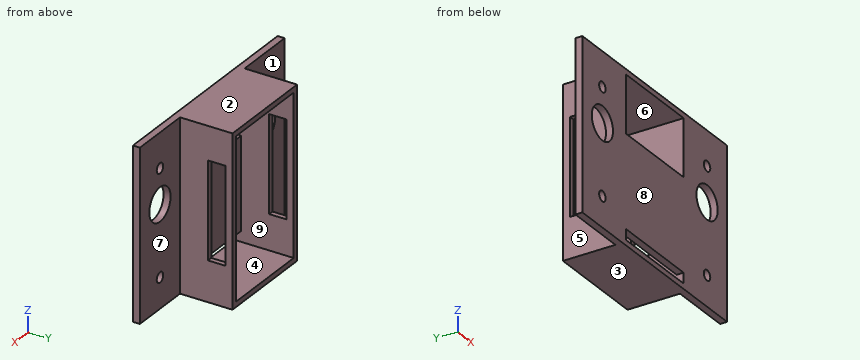
Autodesk Inventor part; units mm, degrees
ref_plane "Work Plane1" through (-23.6, 15, -43.3) normal (0, 1, 0) x (0, 0, 1)
ref_plane "YZ Plane" through (0, 0, 0) normal (1, 0, 0) x (0, 1, 0)
ref_plane "XZ Plane" through (0, 0, 0) normal (0, 1, 0) x (-1, 0, 0)
sketch "Sketch1" plane through (0, 0, 0) normal (0, 1, 0) x (-1, 0, 0)
  line L0 (0, 0) -> (26, 0)
  line L1 (26, 0) -> (26, -45.5)
  line L2 (26, -45.5) -> (0, -45.5)
  line L3 (0, -45.5) -> (0, 0)
  line L4 (-1.5, 0) -> (-1.5, -45.5)
  line L5 (-1.5, -45.5) -> (-1.5, -47)
  line L6 (-1.5, -47) -> (26, -47)
  line L7 (26, -47) -> (27.5, -47)
  line L8 (27.5, -47) -> (27.5, 0)
  line L9 (27.5, 0) -> (27.5, 1.5)
  line L10 (27.5, 1.5) -> (-1.5, 1.5)
  line L11 (-1.5, 1.5) -> (-1.5, 0)
  dimension "d0" = 26
  dimension "d1" = 45.5
  dimension "d3" = 1.5
  dimension "d4" = 1.5
  dimension "d5" = 1.5
extrude "Extrusion1" add sketch "Sketch1" along normal blind 15
sketch "Sketch2" plane through (1.5, 0, 1.5) normal (1, 0, 0) x (0, 0, -1)
  line L0 (9.5, 13) -> (37, 13)
  line L1 (37, 13) -> (37, 8)
  line L2 (9.5, 13) -> (9.5, 8)
  line L3 (37, 8) -> (9.5, 8)
  point P0 (1.5, 0)
  point P1 (48.5, 0)
extrude "Extrusion2" cut sketch "Sketch2" against normal up to surface (29 mm away)
sketch "Sketch3" plane through (0, 0, 0) normal (0, -1, 0) x (1, 0, 0)
  line L0 (1.5, 1.5) -> (1.5, -47)
  line L1 (-27.5, 1.5) -> (1.5, 1.5)
  line L2 (-27.5, -47) -> (-27.5, 1.5)
  line L3 (1.5, -47) -> (-27.5, -47)
  line L4 (0, 0) -> (-26, 0)
  line L5 (0, -45.5) -> (0, 0)
  line L6 (-26, -45.5) -> (0, -45.5)
  line L7 (-26, 0) -> (-26, -45.5)
  line L8 (0, 0) -> (-26, 0)
  line L9 (-26, 0) -> (-26, -3)
  line L10 (-26, 0) -> (-26, -45.5)
  line L11 (-26, -3) -> (0, -3)
  line L12 (0, -45.5) -> (0, 0)
  line L13 (-26, -45.5) -> (-26, -42.5)
  line L14 (-26, -42.5) -> (0, -42.5)
  line L15 (0, -42.5) -> (-26, -42.5)
  line L16 (-26, -42.5) -> (-26, -3)
  line L17 (-26, -3) -> (0, -3)
  line L18 (0, -3) -> (0, -42.5)
  dimension "d15" = 3
  dimension "d16" = 3
extrude "Extrusion3" add sketch "Sketch3" along normal blind 2 contours L0 L3 L2 L1 | L5 L14 L7 L11
sketch "Sketch5" plane through (0, -2, 0) normal (0, -1, 0) x (1, 0, 0)
  line L0 (0, -3) -> (-26, -3)
  line L1 (0, -35.5) -> (0, -8)
  line L2 (-26, -3) -> (0, -3)
  line L3 (0, -3) -> (0, -16.2813)
  line L4 (0, -16.2813) -> (-26, -16.2813)
  line L5 (-26, -16.2813) -> (-26, -3)
  point P0 (0, 0)
  point P1 (0, -8)
ref_plane "Work Plane1" through (-23.6, 15, -43.3) normal (0, 1, 0) x (0, 0, 1)
extrude "Extrusion4" cut sketch "Sketch5" against normal up to surface (17 mm away)
sketch "Sketch6" plane through (1.5, 15, 1.5) normal (1, 0, 0) x (0, 0, -1)
  line L0 (0, -17) -> (48.5, -17)
  line L1 (0, -17) -> (0, -15)
  line L2 (0, 0) -> (0, -17)
  line L3 (0, -15) -> (48.5, -15)
  line L4 (48.5, -17) -> (48.5, 0)
  line L5 (48.5, -17) -> (48.5, -15)
  line L6 (48.5, -17) -> (0, -17)
  point P0 (1.5, -15)
  dimension "d21" = 2
extrude "Extrusion5" add sketch "Sketch6" along normal blind 18
sketch "Sketch7" plane through (-27.5, 15, -47) normal (-1, 0, 0) x (0, 0, 1)
  line L0 (0, -15) -> (48.5, -15)
  line L1 (48.5, -15) -> (48.5, -17)
  line L2 (48.5, -17) -> (0, -17)
  line L3 (0, -17) -> (0, -15)
  point P0 (47, -15)
extrude "Extrusion6" add sketch "Sketch7" along normal blind 18
sketch "Sketch8" plane through (1.5, 0, 1.5) normal (0, 1, 0) x (1, 0, 0)
  circle A0 centre (9, 9.8591) radius 1.4501
  circle A1 centre (9.0001, 39.8592) radius 1.4502
  circle A2 centre (-38, 9.859) radius 1.4499
  circle A3 centre (-38, 39.8587) radius 1.4497
  line L0 (9, 9.8591) -> (9, 19.7911)
  circle A4 centre (9, 19.7911) radius 4.767
  line L1 (-38, 9.859) -> (-38, 19.7911)
  circle A5 centre (-38, 19.7911) radius 4.767
  point P0 (-1.5, 1.5)
  dimension "d26" = 9.932
  dimension "d27" = 9.534
extrude "Extrusion7" cut sketch "Sketch8" against normal up to surface (2 mm away)
properties part number "voltometer_socket"
Geometry: final body of the model. Coordinates: model frame, mm. Face numbers are marked on the shaded views. A direction names the side the tool comes from. Round coordinates to 2 decimals unless told otherwise and drop trailing zeros. Order: outer loops, then holes, each group sorted by start corner. A loop starts at its lowest first (then second) coordinate and runs counter-clockwise, first axis right, second up. Notation, with made-up numbers: (89.5, -20.75) - (119.5, -20.75) arc R15 ccw to (119.5, 4.25) - close; hole circle Ø2 at (49, 46.25). An arc over 180 degrees is marked (long way). Use CSV: the item, a comma, the result in double quotes. Start each with the question number.
Q1. Section query D-D (x = -36.5). Return loops of the section in (y, z).
Q2. Mould query, pull axis Z, two halves, no side actions, for the marked faces 1, 2, 3 and 4. Classes: +Z half, -Z half, draft (parallel to the pull), parting line (faces both ways), or undercut.
Q3. Material intervals for line 1 along Z through (x, y) = (-36.5, -1.6); line 2 along Z through (x, y) = (-16.5, 11); line 3 along X through (y, z) = (4, -5.5), sorted ascending. Write a range as from..to.
Q4. Section query C-C (z = -33). Return loops of the section in (x, y), and give its area (3 significant figures).
Q5. Section query B-B (y = 10). Return loops of the section in (x, z).
Q6. First-contact query: pin 1 (8 mm diameter, centred on y = 12.5, z = -41, fed in from -X); pin 2 (14.5 mm diameter, centred on x = 11, z = -17.5, fed in from +Y); pin 3 (6 mm diameter, centred on y = 5, z = -31, fed in from +X); pin 4 (8.5 mm diameter, centred on x = 10.5, z = -18.29, fed in from +Y). Flat tips, straight axial feed; report the tip coordinate or a pass-through.
Q7. Access query for the marked faces 5, 6, 7, 8 and 9. Directions: +Z, -Z, +X, -X, +Y, -Y. A direction counts if a zero-diameter tool reaches every point of the face in a straight line with its end or side. Return the directions, or none.
Q8. Section query A-A (x = -7). Return loops of the section in (y, z).
Result set:
1,outline,"(-2, -47) - (0, -47) - (0, -39.81) - (-2, -39.81) - close; (-2, -36.91) - (0, -36.91) - (0, -23.06) - (-2, -23.06) - close; (-2, -13.52) - (0, -13.52) - (0, -9.81) - (-2, -9.81) - close; (-2, -6.91) - (0, -6.91) - (0, 1.5) - (-2, 1.5) - close"
2,face 1,"draft"
2,face 2,"+Z half"
2,face 3,"-Z half"
2,face 4,"undercut"
3,line 1,"z = -47..-39.81, -36.91..-23.06, -13.52..-9.81, -6.91..1.5"
3,line 2,"z = -47..-45.5, 0..1.5"
3,line 3,"x = -27.5..-26, 0..1.5"
4,outline,"(-45.5, -2) - (19.5, -2) - (19.5, 0) - (1.5, 0) - (1.5, 8) - (0, 8) - (0, 0) - (-26, 0) - (-26, 8) - (-27.5, 8) - (-27.5, 0) - (-45.5, 0) - close; (-27.5, 13) - (-26, 13) - (-26, 15) - (-27.5, 15) - close; (0, 13) - (1.5, 13) - (1.5, 15) - (0, 15) - close"
4,area,"160 mm2"
5,outline,"(-27.5, -47) - (1.5, -47) - (1.5, -35.5) - (0, -35.5) - (0, -45.5) - (-26, -45.5) - (-26, -35.5) - (-27.5, -35.5) - close; (-27.5, -8) - (-26, -8) - (-26, 0) - (0, 0) - (0, -8) - (1.5, -8) - (1.5, 1.5) - (-27.5, 1.5) - close"
6,pin 1,"stops at x = -27.5"
6,pin 2,"stops at y = 0"
6,pin 3,"stops at x = 1.5"
6,pin 4,"passes through"
7,face 5,"+Z, -Z, -X, +Y"
7,face 6,"+Y, -Y"
7,face 7,"+Z, -Z, +X, +Y"
7,face 8,"+Z, -Z, +X, -X, -Y"
7,face 9,"+Y"
8,outline,"(-2, -47) - (15, -47) - (15, -45.5) - (-2, -45.5) - close; (-2, -42.5) - (0, -42.5) - (0, -16.28) - (-2, -16.28) - close; (-2, 0) - (15, 0) - (15, 1.5) - (-2, 1.5) - close"
